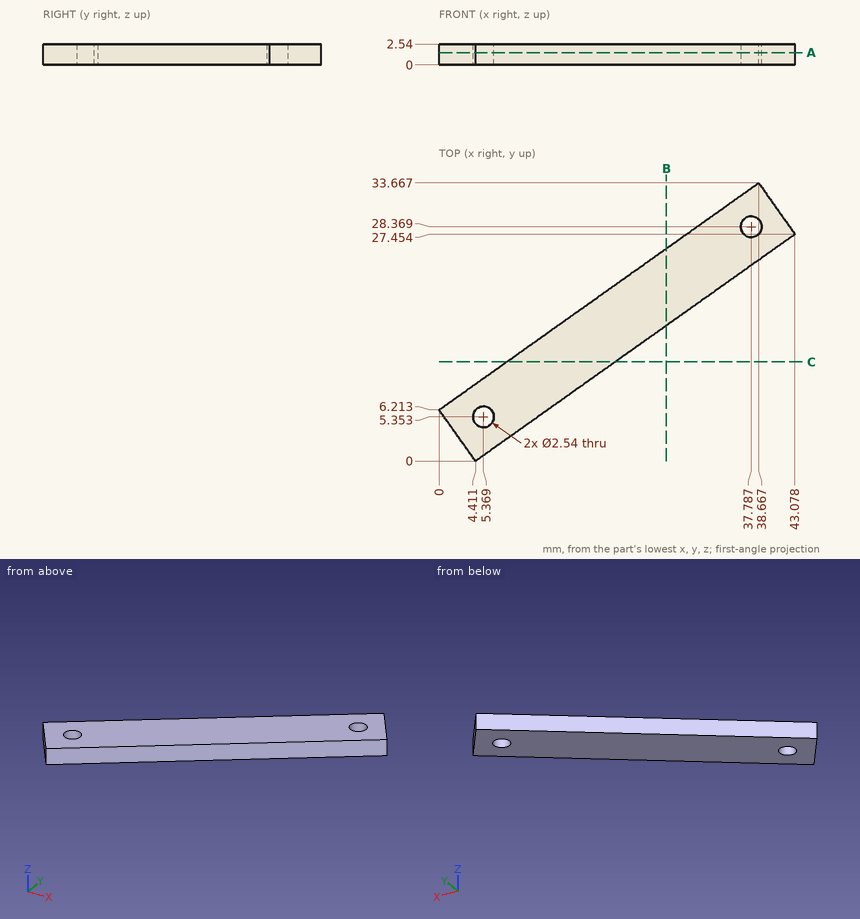
Study the drawing (mm; zero at the part's minimum x, y, z) and answer. Round coordinates to 2 decimals unless told otherwise and drop trailing zeros. Write each loop counter-clockwise with the first axis right and the second up, starting at its lowest first coordinate (ties: lowest second). Pieces come first, ordered by that corner, then holes. Notation, with made-up numbers: (15, -17.5) -> (27, -17.5) arc R21 cw to (27, -11.5) -> close; hole circle Ø11 at (-6.5, -0.5). An arc over 180 degrees is marked (long way). Write item = value, one per line.
1) Section C-C on y = 12 is taken. Write down the section's boundary in (x, z).
Check values:
outline = (8.15, 0) -> (21.31, 0) -> (21.31, 2.54) -> (8.15, 2.54) -> close
2) Section A-A on z = 1.5 is taken. Write down the section's boundary in (x, y), plus the area to 3 significant figures.
Check values:
outline = (0, 6.21) -> (4.41, 0) -> (43.08, 27.45) -> (38.67, 33.67) -> close; hole circle Ø2.54 at (5.37, 5.35); hole circle Ø2.54 at (37.79, 28.37)
area = 351 mm²
3) Straight lines are drawn through the part: line 1 along Y through (x, z) = (37.5, 2.15) (1 decimal); line 2 along X through (y, z) = (6.5, 0.3) (1 decimal); line 3 along Y through (x, z) = (21, 1.4) (1 decimal). For each, find the intervals that lie inside material, in ascending order. Write a range as [from, to].
Check values:
line_1 = [23.5, 27.1], [29.6, 32.8]
line_2 = [0.4, 4.8], [5.9, 13.6]
line_3 = [11.8, 21.1]
4) Section B-B on x = 27.5 is taken. Write down the section's boundary in (y, z).
Check values:
outline = (16.39, 0) -> (25.74, 0) -> (25.74, 2.54) -> (16.39, 2.54) -> close
5) Given pin 1 (2 mm diameter, centred on x = 5.37, y = 5.35, fed in from -Z), flat-ended and moving along its own axis, determine where the tip first touches the part or whether it passes through.
Check values:
pin_1 = through
